Job drawing, mm, ordinate dimensions from the low corner. One solid piece. A direction names the side the tool comes from. Give positions to 0.01 mm unless a question says otherwise; leave off trailing zeros. Order: outer loops, then holes, each group sorted by start corner. A loop starts at its lowest first (then second) coordinate and runs counter-clockwise, first axis right, second up.
1. Slice it at C-C on x = 14.5. List the corners of the cut face in (y, z), and give its area (3 significant figures).
2. Drop flat-ended pins along their axis: pin 1 Ø5 at (x, z) = (37, 38.5) entering from -Y; pin 2 Ø12 at (y, z) = (23.5, 30.5) entering from +X; pin 3 Ø12 at (y, z) = (22, 49.5) entering from -X. Give the stop position or say it passes through.
3. Probe line 1 (X direction, y = 10, z = 13.5); line 2 (Z direction, x = 16, y = 16). List the from-to ranges inside material, lowest first.
4. Slice it at B-B on y = 15. List the corners of the cut face in (x, z), and give its area (3 significant figures).
5. Slice it at D-D on z = 53.5. List the corners of the cut face in (x, y), and give its area (3 significant figures).
6. Which spindle directions (+Z, -Z, +X, -X, +Y, -Y) get a long thin tool onto all of the face, cutting with end or side? Do the marked faces 1 and 2. Say none if no direction does.
7. Slice it at A-A on z = 15. List the corners of the cut face in (x, y).
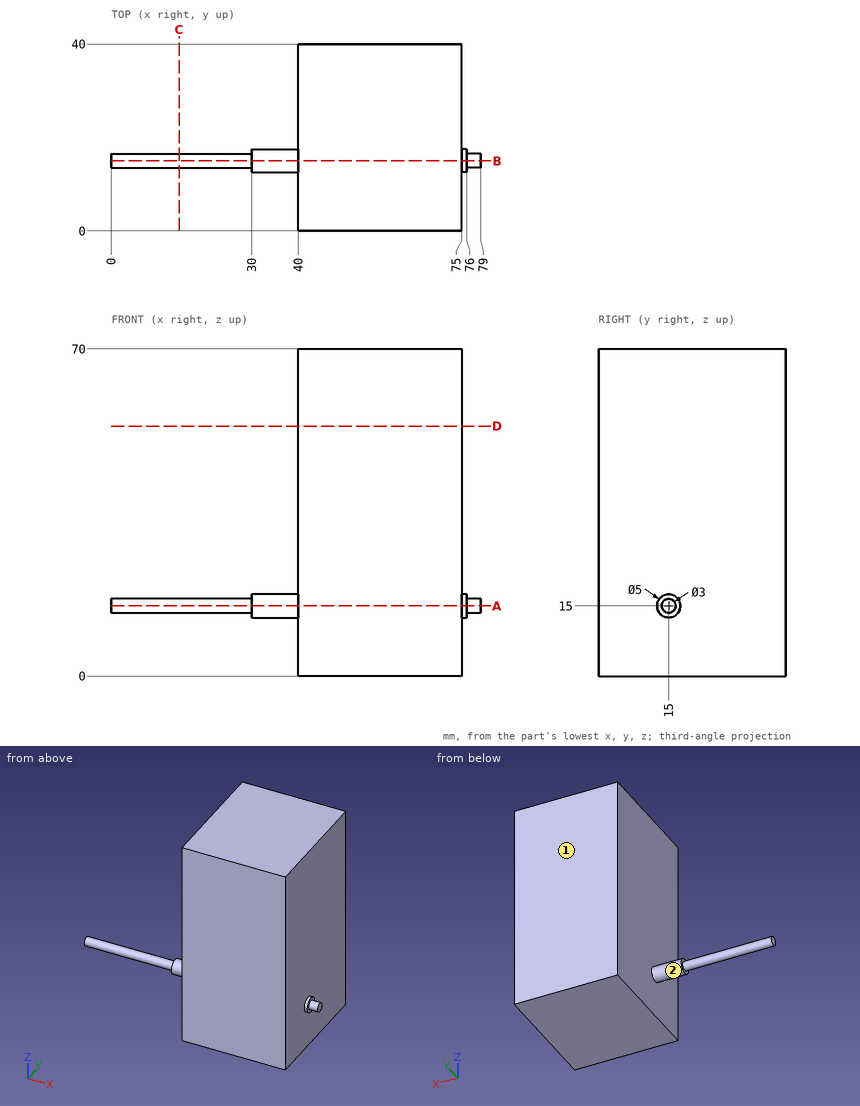
Data:
1. outline: circle Ø3 at (15, 15)
1. area: 7.07 mm2
2. pin 1: passes through
2. pin 2: stops at x = 75
2. pin 3: stops at x = 40
3. line 1: x = 40 to 75
3. line 2: z = 13.88 to 16.12
4. outline: (0, 13.5) - (30, 13.5) - (30, 12.5) - (40, 12.5) - (40, 0) - (75, 0) - (75, 12.5) - (76, 12.5) - (76, 13.5) - (79, 13.5) - (79, 16.5) - (76, 16.5) - (76, 17.5) - (75, 17.5) - (75, 70) - (40, 70) - (40, 17.5) - (30, 17.5) - (30, 16.5) - (0, 16.5) - close
4. area: 2,600 mm2
5. outline: (40, 0) - (75, 0) - (75, 40) - (40, 40) - close
5. area: 1,400 mm2
6. face 1: +Z, -Z, +X, -X, +Y
6. face 2: -X
7. outline: (0, 13.5) - (30, 13.5) - (30, 12.5) - (40, 12.5) - (40, 0) - (75, 0) - (75, 12.5) - (76, 12.5) - (76, 13.5) - (79, 13.5) - (79, 16.5) - (76, 16.5) - (76, 17.5) - (75, 17.5) - (75, 40) - (40, 40) - (40, 17.5) - (30, 17.5) - (30, 16.5) - (0, 16.5) - close
